from build123d import *

# Parameters (mm, degrees)
EXTRUDE_1_DEPTH     = 5
SKETCH_2_R          = 4
EXTRUDE_2_DEPTH     = 8
SKETCH_3_R          = 2.5
EXTRUDE_3_DEPTH     = 1
SKETCH_4_R          = 4
EXTRUDE_4_DEPTH     = 1
SKETCH_5_R          = 2
CUT_EXTRUDE_1_DEPTH = 17.196707484


with BuildPart() as part:
    # 草图1 → 凸台-拉伸1 (new body)
    with BuildSketch(Plane(origin=(0, 0, 0), x_dir=(0, 0, -1), z_dir=(1, 0, 0))):
        Polygon((-2.309401077, 4), (-4.618802154, 0), (-2.309401077, -4), (2.309401077, -4), (4.618802154, 0), (2.309401077, 4), align=None)
    extrude(amount=EXTRUDE_1_DEPTH)

    # 草图2 → 凸台-拉伸2 (add)
    with BuildSketch(Plane(origin=(5, 0, 0), x_dir=(0, 0, -1), z_dir=(1, 0, 0))):
        with Locations(Location((0, 0, 0), (0, 0, 150))):
            Circle(SKETCH_2_R)
    extrude(amount=EXTRUDE_2_DEPTH)

    # 草图3 → 凸台-拉伸3 (add)
    with BuildSketch(Plane(origin=(13, 0, 0), x_dir=(0, 0, -1), z_dir=(1, 0, 0))):
        Circle(SKETCH_3_R)
    extrude(amount=EXTRUDE_3_DEPTH)

    # 草图4 → 凸台-拉伸4 (add)
    with BuildSketch(Plane(origin=(14, 0, 0), x_dir=(0, 0, -1), z_dir=(1, 0, 0))):
        with Locations(Location((0, 0, 0), (0, 0, 150))):
            Circle(SKETCH_4_R)
    extrude(amount=EXTRUDE_4_DEPTH)

    # 草图5 → 切除-拉伸1 (cut, through all)
    with BuildSketch(Plane(origin=(15, 0, 0), x_dir=(0, 0, -1), z_dir=(1, 0, 0))):
        Circle(SKETCH_5_R)
    extrude(amount=-CUT_EXTRUDE_1_DEPTH, mode=Mode.SUBTRACT)


solid = part.part
Can you work these out from the model? Positions are in its coordinate system, mm. A direction names the side the tool comes from. Coordinates: 2 decimals unless noted, no trailing zeros. Write each loop counter-clockwise with the first axis right and the second up, starting at its lowest first coordinate (ties: lowest second). Pieces come first, ordered by that corner, then holes. Notation, with made-up numbers: (3, -23.75) -> (31, -23.75) arc R26 ccw to (31, -7.75) -> close; hole circle Ø6 at (82, 79). An arc over 180 degrees is marked (long way). Write item = value, one per line.
(1) Imagine slicing it at A-A (x = 4.5). Please give me the cut outline in (y, z).
Verdict:
outline = (-4, -2.31) -> (0, -4.62) -> (4, -2.31) -> (4, 2.31) -> (0, 4.62) -> (-4, 2.31) -> close; hole circle Ø4 at (0, 0)
(2) Imagine slicing it at B-B (y = 0.75). Please give me the cut outline in (x, z), and give its area (3 significant figures).
Verdict:
outline = (0, -4.19) -> (5, -4.19) -> (5, -3.93) -> (13, -3.93) -> (13, -2.38) -> (14, -2.38) -> (14, -3.93) -> (15, -3.93) -> (15, -1.85) -> (0, -1.85) -> close; (0, 1.85) -> (15, 1.85) -> (15, 3.93) -> (14, 3.93) -> (14, 2.38) -> (13, 2.38) -> (13, 3.93) -> (5, 3.93) -> (5, 4.19) -> (0, 4.19) -> close
area = 61.7 mm^2
(3) On a 3-axis mill with a long thin cutter (end or side, diameter ignored), from which of +Z, -Z, +X, -X, +Y, -Y can I reach the whole of each face in a straight line? I mean faces 4 (the face through (14.493, -2.15, -3.373)), 5 (the face through (5, 3.6, 2.1)), 6 (the face through (5, 3.6, -2.1)). Say none if no direction works.
Verdict:
face_4 = +X
face_5 = +Z, +X, +Y
face_6 = -Z, +X, +Y
(4) Imagine slicing it at C-C (z = 1). Please give me the cut outline in (x, y).
Verdict:
outline = (0, -4) -> (5, -4) -> (5, -3.87) -> (13, -3.87) -> (13, -2.29) -> (14, -2.29) -> (14, -3.87) -> (15, -3.87) -> (15, -1.73) -> (0, -1.73) -> close; (0, 1.73) -> (15, 1.73) -> (15, 3.87) -> (14, 3.87) -> (14, 2.29) -> (13, 2.29) -> (13, 3.87) -> (5, 3.87) -> (5, 4) -> (0, 4) -> close
(5) Thinking about a two-plate mould opening in X: for faces 1 (the face through (14, 3, -1)), 2 (the face through (5, -3.6, -2.1)), 3 (the face through (2.465, -2.028, -3.448)), which applies, +X half, -X half, draft (parallel to the pull), parting line (faces both ways), or undercut?
Verdict:
face_1 = undercut
face_2 = +X half
face_3 = draft
(6) Imagine slicing it at D-D (y = -3). Please give me the cut outline in (x, z).
Verdict:
outline = (0, -2.89) -> (5, -2.89) -> (5, -2.65) -> (13, -2.65) -> (13, 2.65) -> (5, 2.65) -> (5, 2.89) -> (0, 2.89) -> close; (14, -2.65) -> (15, -2.65) -> (15, 2.65) -> (14, 2.65) -> close
(7) If I drill on probe 1 along X at (y, z) = (-3, -2); probe 2 along Y at (x, z) = (12, -1.25), over which ranges is the centre line in solid material (lowest first)?
Verdict:
probe_1 = 0 to 13, 14 to 15
probe_2 = -3.8 to -1.56, 1.56 to 3.8
(8) For pin 1 (1 mm diameter, centred on x = 2, z = 3, fed in from -Y), with a flat end and sliding along its axis, tell me the tip position at first contact or that it passes through.
Verdict:
pin_1 = -3.67
